```python
from build123d import *

# Parameters (mm, degrees)
F0_W     = 1371.6
F0_H     = 38.1
F1_DEPTH = 38.1
F0_W_2   = 38.1
F0_H_2   = 63.5
F2_DEPTH = 38.1


with BuildPart() as f1:
    # F0 (on Front) → F1 (new body)
    with BuildSketch(Plane.XZ):
        Polygon((-723.9, 76.2), (-723.9, 0), (-685.8, 0), (-685.8, 38.1), (-685.8, 76.2), (-584.037135, 596.9), (-576.591072, 635), (-576.591072, 698.5), (-576.591072, 736.6), (-576.591072, 838.2), (-614.691072, 838.2), (-614.691072, 635), align=None)
        Polygon((-576.591072, 635), (-584.037135, 596.9), (584.037135, 596.9), (576.591072, 635), (322.591072, 635), (284.491072, 635), (-284.491072, 635), (-322.591072, 635), align=None)
        Polygon((576.591072, 736.6), (-576.591072, 736.6), (-576.591072, 698.5), (-322.591072, 698.5), (-284.491072, 698.5), (284.491072, 698.5), (322.591072, 698.5), (576.591072, 698.5), align=None)
        Polygon((685.8, 38.1), (685.8, 0), (723.9, 0), (723.9, 76.2), (614.691072, 635), (614.691072, 838.2), (576.591072, 838.2), (576.591072, 736.6), (576.591072, 698.5), (576.591072, 635), (584.037135, 596.9), (685.8, 76.2), align=None)
        with Locations((0, 57.15)):
            Rectangle(F0_W, F0_H)
        Polygon((-685.8, 0), (-723.9, 0), (-723.9, -38.1), (723.9, -38.1), (723.9, 0), (685.8, 0), align=None)
    extrude(amount=F1_DEPTH)

    # F0 (on Front) → F2 (join)
    with BuildSketch(Plane.XZ):
        Polygon((-723.9, 76.2), (-723.9, 0), (-685.8, 0), (-685.8, 38.1), (-685.8, 76.2), (-584.037135, 596.9), (-576.591072, 635), (-576.591072, 698.5), (-576.591072, 736.6), (-576.591072, 838.2), (-614.691072, 838.2), (-614.691072, 635), align=None)
        Polygon((685.8, 38.1), (685.8, 0), (723.9, 0), (723.9, 76.2), (614.691072, 635), (614.691072, 838.2), (576.591072, 838.2), (576.591072, 736.6), (576.591072, 698.5), (576.591072, 635), (584.037135, 596.9), (685.8, 76.2), align=None)
        Polygon((-685.8, 0), (-723.9, 0), (-723.9, -38.1), (723.9, -38.1), (723.9, 0), (685.8, 0), align=None)
        Polygon((576.591072, 736.6), (-576.591072, 736.6), (-576.591072, 698.5), (-322.591072, 698.5), (-284.491072, 698.5), (284.491072, 698.5), (322.591072, 698.5), (576.591072, 698.5), align=None)
        with Locations((-303.541072, 666.75)):
            Rectangle(F0_W_2, F0_H_2)
        with Locations((303.541072, 666.75)):
            Rectangle(F0_W_2, F0_H_2)
    extrude(amount=F2_DEPTH)


solid = f1.part
```
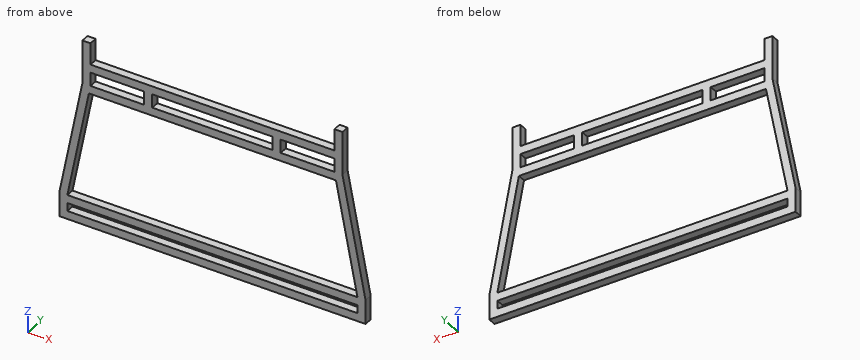
The model under review builds one solid part; all positions refer to its coordinate system, in mm. Give positions to 0.01 mm unless a question says otherwise; leave off trailing zeros. Write each loop counter-clockwise with the first axis right and the second up, starting at its lowest first coordinate (ties: lowest second). Pieces come first, ordered by that corner, then holes.
(1) To check wall thickness, follow L1, parallel to Z at x = -553, y = -27; L2, parallel to X at y = -12, z = 635.5; L3, parallel to X at y = -27, z = 165. State the ranges of each line that lie inside material, in increasing order.
(2) For P1, Ø19, axis at x = -129.5, y = -21, coming from the +Z side; P2, Ø1, axis at y = -31, z = 230.5, coming from the +X side; P3, Ø11.5, axis at y = -11, z = 671.5, coming from the +X side, all flat-tipped, find the tip position at first contact; note any pin that passes through.
(3) Consider section B-B, the plane y = -19. Give the number of separate pieces and of enclosed holes in the cut face, and give its area (3 significant figures).
(4) Consider section D-D, the plane z = 620.5. Give the boundary of the cut face in (x, y).
(5) Consider section C-C, the plane z = 125.5. Give the boundary of the cut face in (x, y).
(6) Consider section A-A, the plane x = 191. Give the boundary of the cut face in (y, z).
Returned:
1. L1: z = -38.1 to 0, 38.1 to 76.2, 596.9 to 635, 698.5 to 736.6
1. L2: x = -614.69 to -576.59, -322.59 to -284.49, 284.49 to 322.59, 576.59 to 614.69
1. L3: x = -706.55 to -668.45, 668.45 to 706.55
2. P1: stops at z = 736.6
2. P2: stops at x = 693.84
2. P3: stops at x = 614.69
3. separate pieces: 1
3. enclosed holes: 5
3. area: 264,000 mm2
4. outline: (-617.52, -38.1) - (617.52, -38.1) - (617.52, 0) - (-617.52, 0) - close
5. outline: (-714.27, -38.1) - (-676.17, -38.1) - (-676.17, 0) - (-714.27, 0) - close; (676.17, -38.1) - (714.27, -38.1) - (714.27, 0) - (676.17, 0) - close
6. outline: (-38.1, -38.1) - (0, -38.1) - (0, 0) - (-38.1, 0) - close; (-38.1, 38.1) - (0, 38.1) - (0, 76.2) - (-38.1, 76.2) - close; (-38.1, 596.9) - (0, 596.9) - (0, 635) - (-38.1, 635) - close; (-38.1, 698.5) - (0, 698.5) - (0, 736.6) - (-38.1, 736.6) - close
